Verification items for the finished model (mm, model axes). Face numbers are marked on the shaded views. A direction names the side the tool comes from. Give positions to 0.01 mm unless a question says otherwise; leave off trailing zeros. Order: outer loops, then holes, each group sorted by start corner. A loop starts at its lowest first (then second) coordinate and runs counter-clockwise, first axis right, second up. Notation, with made-up numbers: (89.5, 77.5) -> (96.5, 77.5) arc R27 ccw to (96.5, 99.5) -> close; hole circle Ø5 at (27.25, -37.5). An arc over 180 degrees is marked (long way). Return JSON: item names as keys, results as strings. Group by question number.
(1) Thickness scan on line 1 along Y through (x, z) = (45.5, 22.5); line 2 along X through (y, z) = (21, 93); line 3 along Y through (x, z) = (-0.5, 66). Record the ranges inside material, lowest first.
(2) Cross-section at B-B on y = 24.5. Enter the section's corners in (x, z), then the cut area to 3 significant figures.
(3) Release check for a two-part mould opening along Y. For the marked faces 3, 4 and 5 record: pulls with the +Y half, pulls with the -Y half, needs draft (parallel to the pull), parting line crosses it, or undercut.
(4) Cross-section at D-D on y = 105. Enter the section's corners in (x, z).
(5) Tool access check on the marked faces 1 and 2. Record the directions out of +Z, -Z, +X, -X, +Y, -Y that give a thin tool (end or side, any length) a straight path to the whole face; none if there is none.
(6) Cross-section at C-C on x = 50.5. Enter the section's corners in (y, z), then the cut area to 3 significant figures.
(7) Depth check by flat-ended pin: pin 1 Ø4 at (x, z) = (46.5, 12) entering from +Y. Enter the tip coordinate at first touch or a pass-through.
(8) Cross-section at A-A on z = 57. Enter the section's corners in (x, y), then the cut area to 3 significant figures.
from build123d import *

# Parameters (mm, degrees)
SKETCH1_W           = 120
SKETCH1_H           = 120
BOSS_EXTRUDE1_DEPTH = 120
FILLET1_R           = 20
SKETCH4_R           = 8.6064573
BOSS_EXTRUDE4_DEPTH = 20
SKETCH5_R           = 2.5
BOSS_EXTRUDE5_DEPTH = 20
FILLET2_R           = 5


with BuildPart() as part:
    # Sketch1 → Boss-Extrude1 (new body)
    with BuildSketch(Plane(origin=(0, 0, 0), x_dir=(1, 0, 0), z_dir=(0, 1, 0))):
        with Locations((54, -46.284032095)):
            Rectangle(SKETCH1_W, SKETCH1_H)
    extrude(amount=BOSS_EXTRUDE1_DEPTH)

    # Fillet1
    fillet1_edges = [part.edges().sort_by_distance(p)[0] for p in [
        (-6, 120, 46.284032095),
        (54, 120, 106.284032095),
        (114, 120, 46.284032095),
        (54, 120, -13.715967905),
        (114, 60, 106.284032095),
        (-6, 60, 106.284032095),
        (-6, 60, -13.715967905),
        (114, 60, -13.715967905),
    ]]
    fillet(fillet1_edges, radius=FILLET1_R)

    # Sketch4 → Boss-Extrude4 (add)
    with BuildSketch(Plane(origin=(0, 120, 0), x_dir=(1, 0, 0), z_dir=(0, 1, 0))):
        with Locations((79.473330559, -18.374712085)):
            Circle(SKETCH4_R)
    extrude(amount=BOSS_EXTRUDE4_DEPTH)

    # Sketch5 → Boss-Extrude5 (add)
    with BuildSketch(Plane(origin=(0, 140, 0), x_dir=(1, 0, 0), z_dir=(0, 1, 0))):
        with Locations((79.473330559, -18.374712085)):
            Circle(SKETCH5_R)
    extrude(amount=BOSS_EXTRUDE5_DEPTH)

    # Fillet2
    fillet2_edges = [part.edges().sort_by_distance(p)[0] for p in [
        (70.866873258, 140, 18.374712085),
    ]]
    fillet(fillet2_edges, radius=FILLET2_R)


solid = part.part
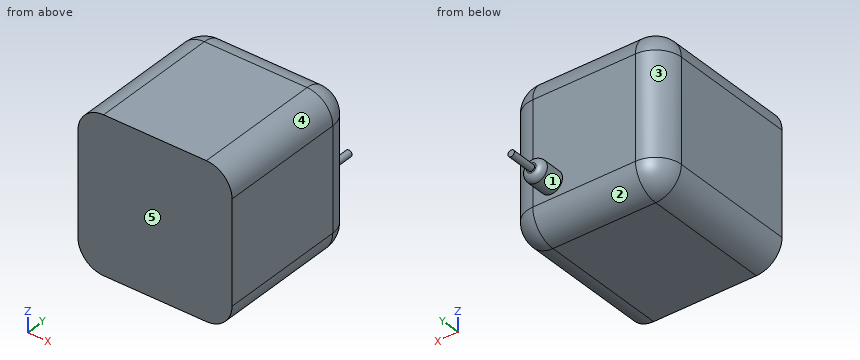
Verdict:
{
 "1": {"line 1": "0 to 120", "line 2": "-4.84 to 112.84", "line 3": "0 to 113.77"},
 "2": {"outline": "(-6, 6.28) arc R20 ccw to (14, -13.72) -> (94, -13.72) arc R20 ccw to (114, 6.28) -> (114, 86.28) arc R20 ccw to (94, 106.28) -> (14, 106.28) arc R20 ccw to (-6, 86.28) -> close", "area": "14,100 mm²"},
 "3": {"face 3": "pulls with the +Y half", "face 4": "needs draft", "face 5": "pulls with the -Y half"},
 "4": {"outline": "(-5.36, 6.28) arc R19.36 ccw to (14, -13.08) -> (94, -13.08) arc R19.36 ccw to (113.36, 6.28) -> (113.36, 86.28) arc R19.36 ccw to (94, 105.65) -> (14, 105.65) arc R19.36 ccw to (-5.36, 86.28) -> close"},
 "5": {"face 1": "+Y", "face 2": "-Z, +X, -X, +Y"},
 "6": {"outline": "(0, -13.72) -> (100, -13.72) arc R20 ccw to (120, 6.28) -> (120, 86.28) arc R20 ccw to (100, 106.28) -> (0, 106.28) -> close", "area": "14,200 mm²"},
 "7": {"pin 1": "y = 120"},
 "8": {"outline": "(-6, 0) -> (114, 0) -> (114, 100) arc R20 ccw to (94, 120) -> (14, 120) arc R20 ccw to (-6, 100) -> close", "area": "14,200 mm²"}
}
